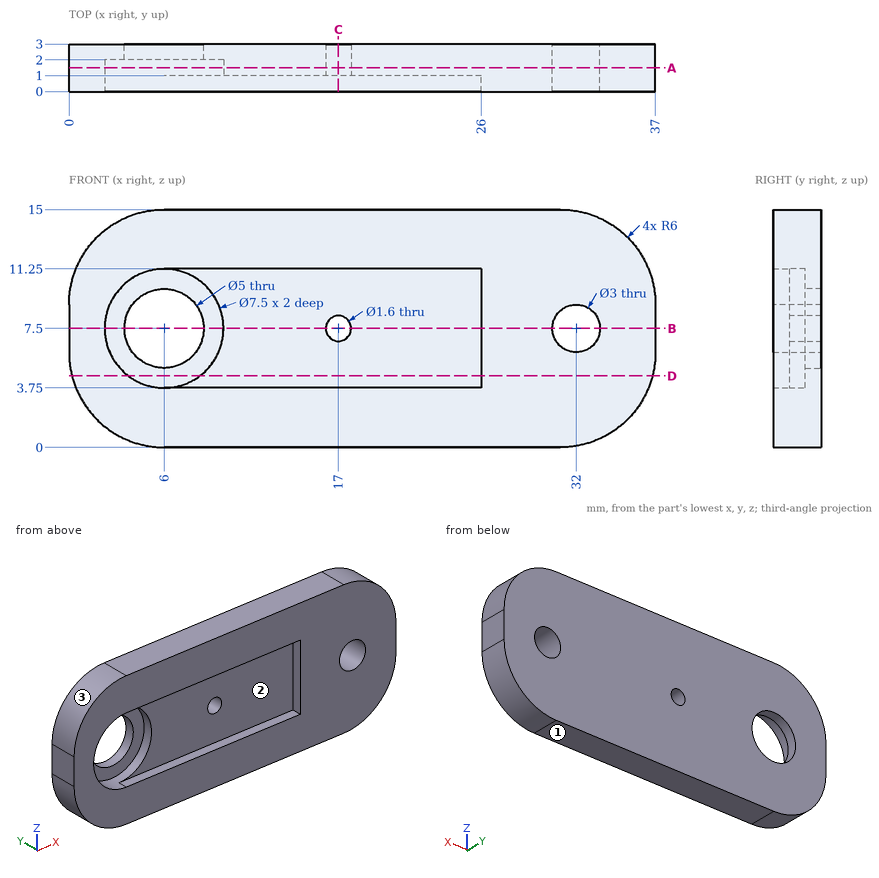
Verification items for this drawing (mm, ordinates from the low corner). Give positions to 0.01 mm unless a question says otherwise; leave off trailing zeros. Write each loop counter-clockwise with the first axis right and the second up, starting at its lowest first coordinate (ties: lowest second). Pieces come first, ordered by that corner, then holes.
1) Release check for a two-part mould opening along Z. For the marked faces 1, 2 and 3 record: pulls with the +Z half, pulls with the -Z half, needs draft (parallel to the pull), parting line crosses it, or undercut.
2) Section check D-D, the plane z = 4.5. Record the boundary of the cut face in (x, y), and give its area (3 significant figures).
3) Section check C-C, the plane x = 17. Record the boundary of the cut face in (y, z), and give its area (3 significant figures).
4) Section check A-A, the plane y = 1.5. Record the boundary of the cut face in (x, z), and give its area (3 significant figures).
5) Section check B-B, the plane z = 7.5. Record the boundary of the cut face in (x, y).
6) Gauge pin test, flat ends, axial feed: pin 1 (0.8 mm diameter, centred on y = 0.5, z = 6, fed in from -X); pin 2 (2.5 mm diameter, centred on x = 17, z = 7.5, fed in from -Y); pin 3 (2 mm diameter, centred on x = 5, z = 9, fed in from -Y). Record the tip position at first contact, or that the pin passes through.
7) Material ranges on L1, parallel to X at y = 2.2, z = 7.5; L2, parallel to X at y = 1.65, z = 7.5; L3, parallel to X at y = 0.65, z = 7.5, recorded low to high.
Computed:
1. face 1: pulls with the -Z half
1. face 2: undercut
1. face 3: pulls with the +Z half
2. outline: (0.19, 0) - (3.75, 0) - (3.75, 2) - (8.25, 2) - (8.25, 1) - (26, 1) - (26, 0) - (36.81, 0) - (36.81, 3) - (0.19, 3) - close
2. area: 83.1 mm2
3. outline: (0, 0) - (3, 0) - (3, 6.7) - (1, 6.7) - (1, 3.75) - (0, 3.75) - close; (0, 11.25) - (1, 11.25) - (1, 8.3) - (3, 8.3) - (3, 15) - (0, 15) - close
3. area: 34.3 mm2
4. outline: (0, 6) arc R6 ccw to (6, 0) - (31, 0) arc R6 ccw to (37, 6) - (37, 9) arc R6 ccw to (31, 15) - (6, 15) arc R6 ccw to (0, 9) - close; hole circle Ø7.5 at (6, 7.5); hole circle Ø1.6 at (17, 7.5); hole circle Ø3 at (32, 7.5)
4. area: 471 mm2
5. outline: (0, 0) - (2.25, 0) - (2.25, 2) - (3.5, 2) - (3.5, 3) - (0, 3) - close; (8.5, 2) - (9.75, 2) - (9.75, 1) - (16.2, 1) - (16.2, 3) - (8.5, 3) - close; (17.8, 1) - (26, 1) - (26, 0) - (30.5, 0) - (30.5, 3) - (17.8, 3) - close; (33.5, 0) - (37, 0) - (37, 3) - (33.5, 3) - close
6. pin 1: stops at x = 0
6. pin 2: stops at y = 1
6. pin 3: stops at y = 2
7. L1: x = 0 to 3.5, 8.5 to 16.2, 17.8 to 30.5, 33.5 to 37
7. L2: x = 0 to 2.25, 9.75 to 16.2, 17.8 to 30.5, 33.5 to 37
7. L3: x = 0 to 2.25, 26 to 30.5, 33.5 to 37
